Could you check a few things on this model? Use its own coordinates, in mm. Face numbers are marked on the shaded views. A direction names the side the tool comes from. Coordinates: 2 decimals unless noted, no trailing zeros. Loops run counter-clockwise (first coordinate to the right, second up) from the corner with the lowest first, then second, coordinate; pieces in that order, holes last. Notation, with made-up numbers: (3, -30) -> (12, -30) arc R15 cw to (12, -25) -> close; hole circle Ø6 at (-38, 76.5). An arc over 180 degrees is marked (long way). One line per question, with ' | ' between items.
```python
from build123d import *

# Parameters (mm, degrees)
F0_W         = 38.1
F0_H         = 107.95
F1_DEPTH     = 6.35
F2_W         = 22.225
F2_H         = 73.025
F3_DEPTH     = 3.175
F4_W         = 38.1
F4_H         = 107.95
F4_W_2       = 31.75
F4_H_2       = 3.175
F5_DEPTH     = 31.75
F6_R         = 15.875
F6_R_2       = 2.5
F7_DEPTH     = 1.5875
F8_R         = 2.5
F9_DEPTH     = 25.4
F10_R        = 8
F11_DEPTH    = 25.4
F12_W        = 9.525
F12_H        = 3.175
F13_DEPTH    = 25.4
F14_W        = 31.75
F14_H        = 3.175
F15_DEPTH    = 3.175
F16_W        = 5.08
F16_H        = 3.175
F17_DEPTH    = 38.1
F18_T1_DEPTH = 134.0782991577


# Not quite as in the source:
# - a fillet or chamfer that OpenCascade refuses, or shapes differently, is made with other operations: its cross-section is extruded or revolved along the edge and cut away or added


with BuildPart() as f1:
    # F0 (on Top) → F1 (new body)
    with BuildSketch(Plane.XY):
        with Locations((19.05, -53.975)):
            Rectangle(F0_W, F0_H)
    extrude(amount=F1_DEPTH)

    # F2 (on face) → F3 (cut)
    with BuildSketch(Plane.XY.offset(6.35)):
        with Locations((19.05, -61.2775)):
            Rectangle(F2_W, F2_H)
    extrude(amount=-F3_DEPTH, mode=Mode.SUBTRACT)

    # F4 (on face) → F5 (join)
    with BuildSketch(Plane.XY.offset(6.35)):
        with Locations((19.05, -53.975)):
            Rectangle(F4_W, F4_H)
        Polygon((3.175, -98.425), (3.175, -3.175), (34.925, -3.175), (34.925, -98.425), (34.925, -101.6), (34.925, -104.775), (3.175, -104.775), (3.175, -101.6), align=None, mode=Mode.SUBTRACT)
        with Locations((19.05, -100.0125)):
            Rectangle(F4_W_2, F4_H_2)
    extrude(amount=F5_DEPTH)

    # F6 (on face) → F7 (cut)
    with BuildSketch(Plane(origin=(0, 0, 0), x_dir=(-1, 0, 0), z_dir=(0, 1, 0))):
        with Locations((-19.05, 19.05)):
            Circle(F6_R)
        with Locations((-23.8125, 19.05)):
            Circle(F6_R_2, mode=Mode.SUBTRACT)
        with Locations((-14.2875, 19.05)):
            Circle(F6_R_2, mode=Mode.SUBTRACT)
    extrude(amount=-F7_DEPTH, mode=Mode.SUBTRACT)

    # F8 (on face) → F9 (cut)
    with BuildSketch(Plane(origin=(0, 0, 0), x_dir=(-1, 0, 0), z_dir=(0, 1, 0))):
        with Locations((-14.2875, 19.05)):
            Circle(F8_R)
        with Locations((-23.8125, 19.05)):
            Circle(F8_R)
    extrude(amount=-F9_DEPTH, mode=Mode.SUBTRACT)

    # F10 (on face) → F11 (cut)
    with BuildSketch(Plane(origin=(0, 0, 0), x_dir=(0, -1, 0), z_dir=(-1, 0, 0))):
        with Locations((13.08, 19.05)):
            Circle(F10_R)
    extrude(amount=-F11_DEPTH, mode=Mode.SUBTRACT)

    # F12 (on face) → F13 (cut)
    with BuildSketch(Plane.XY.offset(6.35)):
        with Locations((19.05, -103.1875)):
            Rectangle(F12_W, F12_H)
    extrude(amount=-F13_DEPTH, mode=Mode.SUBTRACT)

    # F14 (on face) → F15 (cut)
    with BuildSketch(Plane.XY.offset(38.1)):
        with Locations((19.05, -100.0125)):
            Rectangle(F14_W, F14_H)
    extrude(amount=-F15_DEPTH, mode=Mode.SUBTRACT)

    # F16 (on face) → F17 (join)
    with BuildSketch(Plane.YZ.offset(38.1)):
        with Locations((-5.715, 33.3375)):
            Rectangle(F16_W, F16_H)
    extrude(amount=-F17_DEPTH)

    # F18: chamfer of 5.08 on 4 edges, made by hand

    # F18_s2 → F18_t1 (cut)
    with BuildSketch(Plane.XZ.offset(-13.0641495789)):
        Polygon((38.1, 5.08), (33.02, 0), (38.1, 0), align=None)
        Polygon((38.1, 33.02), (33.02, 38.1), (38.1, 38.1), align=None)
        Polygon((5.08, 38.1), (0, 33.02), (0, 38.1), align=None)
        Polygon((5.08, 0), (0, 5.08), (0, 0), align=None)
    extrude(amount=F18_T1_DEPTH, mode=Mode.SUBTRACT)


solid = f1.part
```
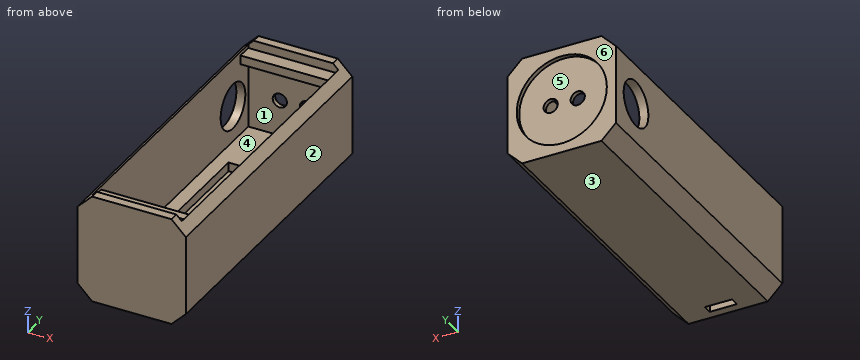
Q1. Please list where these lines run through material, in increasing order: L1, parallel to Y at x = 5.5, z = 29.5 (3 decimals); L2, parallel to X at y = -2, z = 19; L3, parallel to Y at x = 2, z = 19. Write a range as [from, to].
Values follow:
L1: y = [-107.95, -104.775], [-101.6, -98.425], [-3.175, 0] | L2: x = [0, 11.79], [16.79, 21.31], [26.31, 38.1] | L3: y = [-107.95, -21.08], [-5.08, 0]
Q2. For the marked faces 1 and 2, which set-ups out of +Z, -Z, +X, -X, +Y, -Y let a thin tool reach every point of the face, with its end or its side?
Values follow:
face 1: none | face 2: +Z, -Z, +X, +Y, -Y
Q3. We'd pull the mould along Z, two halves only. Please class the marked faces 3, 4, 5 and 6: released by +Z, released by -Z, zero draft, split by the parting line, or undercut.
Values follow:
face 3: released by -Z | face 4: undercut | face 5: undercut | face 6: zero draft
Q4. Imagine slicing it at C-C on y = -13.08. Write out the boundary of the cut face in (x, z) (3 decimals).
Values follow:
outline: (0, 5.08) -> (5.08, 0) -> (33.02, 0) -> (38.1, 5.08) -> (38.1, 33.02) -> (34.925, 36.195) -> (34.925, 6.35) -> (3.175, 6.35) -> (3.175, 11.05) -> (0, 11.05) -> close; (0, 27.05) -> (3.175, 27.05) -> (3.175, 36.195) -> (0, 33.02) -> close
Q5. For pin 1 (3.5 mm diameter, centred on y = -102.5, z = 2.5, fed in from -X); pin 2 (5 mm diameter, centred on x = 6.5, y = -43.5, fed in from +Z); pin 3 (9.5 mm diameter, centred on x = 12.5, z = 16, fed in from +Y), each with a flat end and sliding along its axis, tell me the tip position at first contact or that it passes through.
Values follow:
pin 1: stops at x = 0.83 | pin 2: stops at z = 6.35 | pin 3: stops at y = -1.59
Q6. Imagine slicing it at A-A on z = 19.05. Give the number of separate pieces and of enclosed holes in the cut face, plus the area to 3 significant figures.
Values follow:
separate pieces: 3 | enclosed holes: 1 | area: 871 mm2
